from build123d import *

# Parameters (mm, degrees)
SKETCH1_W                                       = 200
SKETCH1_H                                       = 50
BOSS_EXTRUDE1_DEPTH                             = 25
CBORE_FOR_M8_SOCKET_HEAD_CAP_SCREW1_D           = 9
CBORE_FOR_M8_SOCKET_HEAD_CAP_SCREW1_CBORE_D     = 14
CBORE_FOR_M8_SOCKET_HEAD_CAP_SCREW1_CBORE_DEPTH = 9


with BuildPart() as part:
    # Sketch1 → Boss-Extrude1 (new body)
    with BuildSketch(Plane(origin=(0, 0, 0), x_dir=(0, 0, -1), z_dir=(1, 0, 0))):
        with Locations((0, 25)):
            Rectangle(SKETCH1_W, SKETCH1_H)
    extrude(amount=BOSS_EXTRUDE1_DEPTH)

    # CBORE for M8 Socket Head Cap Screw1 (through all)
    with Locations(Plane(origin=(0, 50, 0), x_dir=(-1, 0, 0), z_dir=(0, 1, 0))):
        with Locations((-12.5, 80), (-12.5, -80)):
            CounterBoreHole(CBORE_FOR_M8_SOCKET_HEAD_CAP_SCREW1_D / 2, CBORE_FOR_M8_SOCKET_HEAD_CAP_SCREW1_CBORE_D / 2, CBORE_FOR_M8_SOCKET_HEAD_CAP_SCREW1_CBORE_DEPTH)


solid = part.part
Geometry: final body of the model. Coordinates: model frame, mm. A direction names the side the tool comes from. Round coordinates to 2 decimals unless told otherwise and drop trailing zeros. Loops run counter-clockwise (first coordinate to the right, second up) from the corner with the lowest first, then second, coordinate; pieces in that order, holes last.
Q1. Material intervals for L1, parallel to Z at x = 12.5, y = 46.75; L2, parallel to Z at x = 12.5, y = 32, sorted ascending.
Q2. Section C-C on y = 27.5. Return loops of the section in (x, z), plus the area to 3 significant figures.
Q3. Section A-A on z = -80. Return loops of the section in (x, y), plus the area to 3 significant figures.
Q4. Section B-B on x = 12.5. Return loops of the section in (y, z).
Q5. Pin query (flat end, axial travel): P1, Ø1.5, axis at x = 5, z = 44, coming from the -Y side; P2, Ø11, axis at x = 12.5, z = -81, coming from the +Y side. Return the tip coordinate at first contact, or that it passes through.
Q6. Access query for faces 1 (the flat face through (12, 25, -100)), 2 (the flat face through (13, 41, -85)). Directions: +Z, -Z, +X, -X, +Y, -Y. A direction counts if a zero-diameter tool reaches every point of the face in a straight line with its end or side. Return the directions, or none.
Q7. Pull-direction query (Z, two-part tool) for faces 3 (the cylindrical face through (11.91, 20.21, -75.54)), 4 (the flat face through (12, 25, 100)), 5 (the flat face through (25, 25, 1)); classes: released by +Z, released by -Z, zero draft, split by the parting line, or undercut.
Q8. Section D-D on y = 45.5. Return loops of the section in (x, z).
Evaluation:
1. L1: z = -100 to -87, -73 to 73, 87 to 100
1. L2: z = -100 to -84.5, -75.5 to 75.5, 84.5 to 100
2. outline: (0, -100) - (25, -100) - (25, 100) - (0, 100) - close; hole circle Ø9 at (12.5, -80); hole circle Ø9 at (12.5, 80)
2. area: 4,870 mm2
3. outline: (0, 0) - (8, 0) - (8, 41) - (5.5, 41) - (5.5, 50) - (0, 50) - close; (17, 0) - (25, 0) - (25, 50) - (19.5, 50) - (19.5, 41) - (17, 41) - close
3. area: 755 mm2
4. outline: (0, -100) - (50, -100) - (50, -87) - (41, -87) - (41, -84.5) - (0, -84.5) - close; (0, -75.5) - (41, -75.5) - (41, -73) - (50, -73) - (50, 73) - (41, 73) - (41, 75.5) - (0, 75.5) - close; (0, 84.5) - (41, 84.5) - (41, 87) - (50, 87) - (50, 100) - (0, 100) - close
5. P1: stops at y = 0
5. P2: stops at y = 41
6. face 1: -Z, +X, -X, +Y, -Y
6. face 2: +Y
7. face 3: undercut
7. face 4: released by +Z
7. face 5: zero draft
8. outline: (0, -100) - (25, -100) - (25, 100) - (0, 100) - close; hole circle Ø14 at (12.5, -80); hole circle Ø14 at (12.5, 80)
